```python
from build123d import *

# Parameters (mm, degrees)
SKETCH1_R           = 3
SKETCH1_R_2         = 2.5
SKETCH1_R_3         = 20
BOSS_EXTRUDE1_DEPTH = 12
CUT_EXTRUDE1_DEPTH  = 6


with BuildPart() as part:
    # Sketch1 → Boss-Extrude1 (new body)
    with BuildSketch(Plane(origin=(0, 0, 0), x_dir=(1, 0, 0), z_dir=(0, 1, 0))):
        with BuildLine():
            Line((10, 0), (100, 0))
            ThreePointArc((100, 0), (107.071067812, 2.928932188), (110, 10))
            Line((110, 10), (110, 50))
            Line((110, 50), (90, 50))
            Line((90, 50), (90, 60))
            Line((90, 60), (110, 60))
            Line((110, 60), (110, 65))
            ThreePointArc((110, 65), (107.071067812, 72.071067812), (100, 75))
            Line((100, 75), (10, 75))
            ThreePointArc((10, 75), (2.928932188, 72.071067812), (0, 65))
            Line((0, 65), (0, 60))
            Line((0, 60), (20, 60))
            Line((20, 60), (20, 50))
            Line((20, 50), (0, 50))
            Line((0, 50), (0, 10))
            ThreePointArc((0, 10), (2.928932188, 2.928932188), (10, 0))
        make_face()
        with Locations(Location((15, 20, 0), (0, 0, 270))):
            Circle(SKETCH1_R, mode=Mode.SUBTRACT)
        with Locations(Location((78.5, 56, 0), (0, 0, 270))):
            Circle(SKETCH1_R_2, mode=Mode.SUBTRACT)
        with Locations(Location((95, 20, 0), (0, 0, 90))):
            Circle(SKETCH1_R, mode=Mode.SUBTRACT)
        with Locations(Location((55, 32.5, 0), (0, 0, 270))):
            Circle(SKETCH1_R_3, mode=Mode.SUBTRACT)
        with Locations(Location((31.5, 56, 0), (0, 0, 90))):
            Circle(SKETCH1_R_2, mode=Mode.SUBTRACT)
        with Locations(Location((78.5, 9, 0), (0, 0, 90))):
            Circle(SKETCH1_R_2, mode=Mode.SUBTRACT)
        with Locations(Location((31.5, 9, 0), (0, 0, 270))):
            Circle(SKETCH1_R_2, mode=Mode.SUBTRACT)
    extrude(amount=BOSS_EXTRUDE1_DEPTH)

    # Sketch2 → Cut-Extrude1 (cut)
    with BuildSketch(Plane.XZ):
        Polygon((29.046261356, -51.75), (26.592522712, -56), (29.046261356, -60.25), (33.953738644, -60.25), (36.407477288, -56), (33.953738644, -51.75), align=None)
        Polygon((76.046261356, -51.75), (73.592522712, -56), (76.046261356, -60.25), (80.953738644, -60.25), (83.407477288, -56), (80.953738644, -51.75), align=None)
    extrude(amount=-CUT_EXTRUDE1_DEPTH, mode=Mode.SUBTRACT)


solid = part.part
```
Geometry: final body of the model. Coordinates: model frame, mm. A direction names the side the tool comes from. Round coordinates to 2 decimals unless told otherwise and drop trailing zeros. Order: outer loops, then holes, each group sorted by start corner. A loop starts at its lowest first (then second) coordinate and runs counter-clockwise, first axis right, second up. Notation, with made-up numbers: (33.5, 73.25) -> (84.5, 73.25) arc R23 cw to (84.5, 107.25) -> close; hole circle Ø10 at (77, -30.75). An arc over 180 degrees is marked (long way). Use one line per item in the form item = value.
(1) Access query for faces 1 (the face through (106.99, 5.92, -2.85)), 2 (the face through (12.07, 5.92, -20.65)), 3 (the face through (10, 6, -60)), 4 (the face through (90, 6, -55)), 5 (the face through (74.802, 2.958, -58.095)). Directions: +Z, -Z, +X, -X, +Y, -Y. A direction counts if a zero-diameter tool reaches every point of the face in a straight line with its end or side. Return the directions, or none.
Results list:
face_1 = +Z, +X, +Y, -Y
face_2 = +Y, -Y
face_3 = -X, +Y, -Y
face_4 = +X, +Y, -Y
face_5 = -Y
(2) Section C-C on y = 3. Count the separate pieces of the cut face and the enclosed holes in it, and give its area (3 significant figures).
Results list:
separate_pieces = 1
enclosed_holes = 7
area = 6,290 mm^2
(3) Section B-B on z = -32.5. Return loops of the section in (x, y), and give its area (3 significant figures).
Results list:
outline = (0, 0) -> (35, 0) -> (35, 12) -> (0, 12) -> close; (75, 0) -> (110, 0) -> (110, 12) -> (75, 12) -> close
area = 840 mm^2
(4) Section A-A on x = 78.5. Return loops of the section in (y, z), and give its area (3 significant figures).
Results list:
outline = (0, -75) -> (12, -75) -> (12, -58.5) -> (6, -58.5) -> (6, -60.25) -> (0, -60.25) -> close; (0, -51.75) -> (6, -51.75) -> (6, -53.5) -> (12, -53.5) -> (12, -11.5) -> (0, -11.5) -> close; (0, -6.5) -> (12, -6.5) -> (12, 0) -> (0, 0) -> close
area = 759 mm^2
(5) Draft query along Z for faces 6 (the face through (10, 6, -50)), 7 (the face through (107.15, 5.92, -71.99)), 8 (the face through (110, 6, -30)). Return one class per face: pulls with the +Z half, pulls with the -Z half, needs draft (parallel to the pull), parting line crosses it, or undercut.
Results list:
face_6 = undercut
face_7 = pulls with the -Z half
face_8 = needs draft
(6) Section D-D on x = 55. Return loops of the section in (y, z), and give its area (3 significant figures).
Results list:
outline = (0, -75) -> (12, -75) -> (12, -52.5) -> (0, -52.5) -> close; (0, -12.5) -> (12, -12.5) -> (12, 0) -> (0, 0) -> close
area = 420 mm^2
(7) First-contact query: pin 1 Ø5 at (y, z) = (3.5, -56) entering from -X; pin 2 Ø8 at (x, z) = (95, -20) entering from +Y; pin 3 Ø6 at (x, z) = (78.5, -56) entering from -Y. Flat tips, straight axial feed; report the tip coordinate or a pass-through.
Results list:
pin_1 = 20
pin_2 = 12
pin_3 = 6
(8) Ray query, probe 1 along Z at (x, y) = (78.5, 7.75); probe 2 along X at (y, z) = (10.1, -56); probe 3 along X at (y, z) = (9.25, -9). Return the intervals inside material, ascending. Write a range as [from, to].
Results list:
probe_1 = [-75, -58.5], [-53.5, -11.5], [-6.5, 0]
probe_2 = [20, 29], [34, 76], [81, 90]
probe_3 = [0.05, 29], [34, 76], [81, 109.95]
